Autodesk Inventor part; units mm, degrees
ref_plane "YZ Plane" through (0, 0, 0) normal (1, 0, 0) x (0, 1, 0)
ref_plane "XZ Plane" through (0, 0, 0) normal (0, 1, 0) x (-1, 0, 0)
ref_plane "XY Plane" through (0, 0, 0) normal (0, 0, 1) x (1, 0, 0)
sketch "スケッチ1" plane through (0, 0, 0) normal (0, 0, 1) x (1, 0, 0)
  circle A0 centre (0, 0) radius 15.6
  dimension "d0" = 31.2
extrude "押し出し1" add sketch "スケッチ1" along normal blind 10
sketch "スケッチ2" plane through (0, 0, 10) normal (0, 0, 1) x (1, 0, 0)
  circle A0 centre (0, 0) radius 15.6
  circle A1 centre (0, 0) radius 19.5
  dimension "d3" = 39
extrude "押し出し2" add sketch "スケッチ2" along normal blind 10 contours A0 | A1
chamfer "面取り1" distance 2 angle 45 1 edges at (-15.6, 0, 0)
chamfer "面取り2" distance 0.5 angle 45 2 edges at (-19.5, 0, 20) (-19.5, 0, 10)
sketch "スケッチ3" plane through (0, 0, 20) normal (0, 0, 1) x (1, 0, 0)
  circle A0 centre (0, 0) radius 19
  circle A1 centre (0, 0) radius 11.05
  dimension "d12" = 22.1
extrude "押し出し3" cut sketch "スケッチ3" against normal through all contours A1
chamfer "面取り3" distance 1 angle 45 1 edges at (-11.05, 0, 20)
properties part number "Print_Parts_A3" material "PC/ABS プラスチック"
Check sheet for the modelled part. Datum: model origin and axes. Units: mm. A direction names the side the tool comes from. Round coordinates to 2 decimals unless told otherwise and drop trailing zeros. Write each loop counter-clockwise with the first axis right and the second up, starting at its lowest first coordinate (ties: lowest second). Pieces come first, ordered by that corner, then holes. Notation, with made-up numbers: (-31.5, 73.25) -> (23.5, 73.25) arc R33 cw to (23.5, 106.25) -> close; hole circle Ø2 at (30.25, -0.75). An arc over 180 degrees is marked (long way). One line per question, with ' | ' between items. Start each with the question number.
1. Depth check by flat-ended pin: pin 1 (8 mm diameter, centred on y = -12, z = 15, fed in from +X); pin 2 (6 mm diameter, centred on x = 6.5, z = 8, fed in from -Y); pin 3 (8 mm diameter, centred on x = 15, z = 16.5, fed in from +Y); pin 4 (17.5 mm diameter, centred on x = 0, y = 0, fed in from +Z). Enter the tip coordinate at first touch or a pass-through.
2. Scan lines: line 1 along Y through (x, z) = (0, 10.75); line 2 along Y through (x, z) = (0, 5.5); line 3 along Z through (x, y) = (2, -17). Record each from-to range of solid material in increasing order. Write a range as from..to.
3. Sectioned sample at A-A, the plane y = 0. Record the cut outline in (x, z), then the cut area to 4 significant figures.
4. Sectioned sample at C-C, the plane z = 11. Record the cut outline in (x, y).
5. Release check for a two-part mould opening along Y. For faces 3 (the face through (-2.395, -10.787, 9.633)), 4 (the face through (-2.1, 11.1, 0)), 5 (the face through (-2.98, -13.4, 0.13)) record: +Y half, -Y half, draft (parallel to the pull), parting line (faces both ways), or undercut.
6. Set-up check for faces 1 (the face through (-2.539, -19.334, 14.937)), 2 (the face through (-11.5, -10.54, 5.94)): record each of +Z, -Z, +X, -X, +Y, -Y from which the full face is reachable in a straight line by a thin tool's end or side.
Taken from the geometry:
1) pin 1: stops at x = 17.78 | pin 2: stops at y = -18.89 | pin 3: stops at y = 16.1 | pin 4: passes through
2) line 1: y = -19.5..-11.05, 11.05..19.5 | line 2: y = -15.6..-11.05, 11.05..15.6 | line 3: z = 10..20
3) outline: (-19.5, 10.5) -> (-19, 10) -> (-15.6, 10) -> (-15.6, 2) -> (-13.6, 0) -> (-11.05, 0) -> (-11.05, 19) -> (-12.05, 20) -> (-19, 20) -> (-19.5, 19.5) -> close; (11.05, 0) -> (13.6, 0) -> (15.6, 2) -> (15.6, 10) -> (19, 10) -> (19.5, 10.5) -> (19.5, 19.5) -> (19, 20) -> (12.05, 20) -> (11.05, 19) -> close | area: 254.5 mm^2
4) outline: circle Ø39 at (0, 0); hole circle Ø22.1 at (0, 0)
5) face 3: undercut | face 4: draft | face 5: parting line
6) face 1: +Z, -Z | face 2: -Z
